For this review, take the finished solid that the model builds, in its own axes (mm). Give positions to 0.01 mm unless a question says otherwise; leave off trailing zeros. Write each loop counter-clockwise with the first axis right and the second up, starting at its lowest first coordinate (ties: lowest second). Pieces come first, ordered by that corner, then holes. Notation, with made-up numbers: M -35.5,32.5 L -10.5,32.5 A16 cw -10.5,44.5 Z; hole C 46,31.25 d7. An arc over 180 degrees is marked long. Use one line per item in the form item = value. Start each with the question number.
Q1. Consider section B-B on x = 8.75. Write out the cut boundary in (y, z).
Q2. For probe 1 along X at (y, z) = (1.5, 46); probe 2 along Z at (x, y) = (8.75, 0), list the stretches that pass through material, from the lowest coordinate up. Write a range as [from, to].
Q3. Consider section A-A on z = 46. Write out the cut boundary in (x, y), and give its area (3 significant figures).
Q4. Clearance check with flat-ended pins moving along their axes: pin 1 Ø3.5 at (x, z) = (0, 46) entering from +Y; pin 2 Ø1.9 at (x, z) = (8.75, -45.18) entering from +Y. State where each tip first meets the part, or that it passes through.
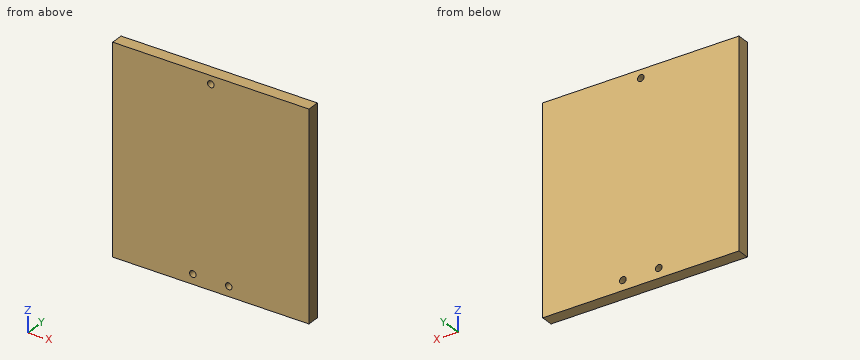
```python
from build123d import *

# Parameters (mm, degrees)
SKETCH1_W           = 95.7
SKETCH1_H           = 100
SKETCH1_R           = 1.6
BOSS_EXTRUDE1_DEPTH = 3


with BuildPart() as part:
    # Sketch1 → Boss-Extrude1 (new body, symmetric)
    with BuildSketch(Plane(origin=(0, 0, 0), x_dir=(1, 0, 0), z_dir=(0, 1, 0))):
        Rectangle(SKETCH1_W, SKETCH1_H)
        with Locations((-8.75, 45.181367204)):
            Circle(SKETCH1_R, mode=Mode.SUBTRACT)
        with Locations((8.75, 45.181367204)):
            Circle(SKETCH1_R, mode=Mode.SUBTRACT)
        with Locations((0, -46)):
            Circle(SKETCH1_R, mode=Mode.SUBTRACT)
    extrude(amount=BOSS_EXTRUDE1_DEPTH, both=True)


solid = part.part
```
Working result:
q1.outline = M -3,-50 L 3,-50 L 3,-46.78 L -3,-46.78 Z; M -3,-43.58 L 3,-43.58 L 3,50 L -3,50 Z
q2.probe_1 = [-47.85, -1.6], [1.6, 47.85]
q2.probe_2 = [-50, -46.78], [-43.58, 50]
q3.outline = M -47.85,-3 L -1.6,-3 L -1.6,3 L -47.85,3 Z; M 1.6,-3 L 47.85,-3 L 47.85,3 L 1.6,3 Z
q3.area = 555 mm²
q4.pin_1 = 3
q4.pin_2 = through
